Build history of the part. All positions in model axes, mm. Coordinates: 2 decimals unless noted, no trailing zeros. Loops run counter-clockwise (first coordinate to the right, second up) from the corner with the lowest first, then second, coordinate; pieces in that order, holes last.
(1) Wall check: L1, parallel to Y at x = -1.5, z = 0.15; L2, parallel to X at y = 2, z = 0.15; L3, parallel to X at y = -3, z = 0.5. Give the ranges that are in metal, low to high.
(2) Slice it at A-A (y = 2.25). Give the cut face in (x, z).
(3) Slice it at D-D (x = -7). Give the cut face in (y, z), and give its area (3 significant figures).
(4) Slice it at C-C (y = -1.75). Give the cut face in (x, z).
(5) Slice it at B-B (z = 0.35). Give the cut face in (x, y).
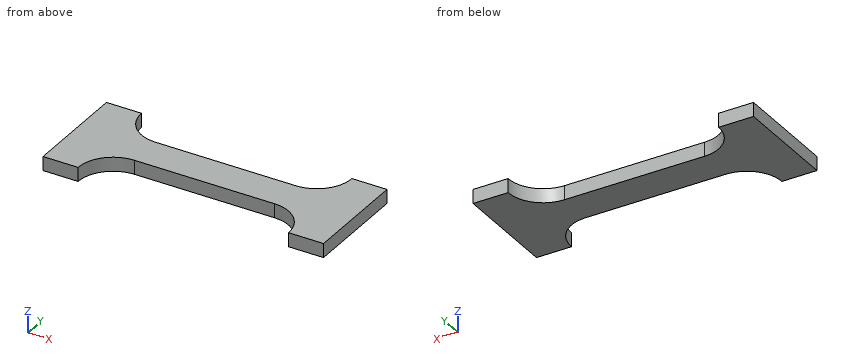
from build123d import *

# Parameters (mm, degrees)
F1_DEPTH = 1


with BuildPart() as f1:
    # F0 (on Top) → F1 (new body)
    with BuildSketch(Plane.XY):
        with BuildLine():
            Line((0, -1.25), (0, 1.25))
            Line((0, 1.25), (-5, 1.25))
            ThreePointArc((-5, 1.25), (-6.767767, 1.982233), (-7.5, 3.75))
            Line((-7.5, 3.75), (-10, 3.75))
            Line((-10, 3.75), (-10, -3.75))
            Line((-10, -3.75), (-7.5, -3.75))
            ThreePointArc((-7.5, -3.75), (-6.767767, -1.982233), (-5, -1.25))
            Line((-5, -1.25), (0, -1.25))
        make_face()
        with BuildLine():
            ThreePointArc((7.5, 3.75), (6.767767, 1.982233), (5, 1.25))
            Line((5, 1.25), (0, 1.25))
            Line((0, 1.25), (0, -1.25))
            Line((0, -1.25), (5, -1.25))
            ThreePointArc((5, -1.25), (6.767767, -1.982233), (7.5, -3.75))
            Line((7.5, -3.75), (10, -3.75))
            Line((10, -3.75), (10, 3.75))
            Line((10, 3.75), (7.5, 3.75))
        make_face()
    extrude(amount=F1_DEPTH)


solid = f1.part
Response values:
1. L1: y = -1.25 to 1.25
1. L2: x = -10 to -6.79, 6.79 to 10
1. L3: x = -10 to -7.38, 7.38 to 10
2. outline: (-10, 0) - (-7, 0) - (-7, 1) - (-10, 1) - close; (7, 0) - (10, 0) - (10, 1) - (7, 1) - close
3. outline: (-2.25, 0) - (2.25, 0) - (2.25, 1) - (-2.25, 1) - close
3. area: 4.50 mm2
4. outline: (-10, 0) - (-6.5, 0) - (-6.5, 1) - (-10, 1) - close; (6.5, 0) - (10, 0) - (10, 1) - (6.5, 1) - close
5. outline: (-10, -3.75) - (-7.5, -3.75) arc R2.5 cw to (-5, -1.25) - (5, -1.25) arc R2.5 cw to (7.5, -3.75) - (10, -3.75) - (10, 3.75) - (7.5, 3.75) arc R2.5 cw to (5, 1.25) - (-5, 1.25) arc R2.5 cw to (-7.5, 3.75) - (-10, 3.75) - close
